Part model, mm, in its own coordinate system. A direction names the side the tool comes from. Round coordinates to 2 decimals unless told otherwise and drop trailing zeros. Order: outer loops, then holes, each group sorted by start corner. A loop starts at its lowest first (then second) coordinate and runs counter-clockwise, first axis right, second up. Notation, with made-up numbers: (89.5, -16.75) -> (134.5, -16.75) arc R29 ccw to (134.5, 4.25) -> close; hole circle Ø8 at (-7, 64.5). An arc over 180 degrees is marked (long way). Answer as a JSON object with one key per item and string values. Group by question number.
```python
from build123d import *

# Parameters (mm, degrees)
F0_W     = 105
F0_H     = 85
F0_W_2   = 72
F0_H_2   = 40
F1_ANGLE = 48


with BuildPart() as f1:
    # F0 (on Front) → F1 (revolve)
    with BuildSketch(Plane.XZ):
        Rectangle(F0_W, F0_H)
        with Locations((0, 12.5)):
            Rectangle(F0_W_2, F0_H_2, mode=Mode.SUBTRACT)
    revolve(axis=Axis((0, 0, -42.5), (-1, 0, 0)), revolution_arc=F1_ANGLE)


solid = f1.part
```
Q1. Band-saw the part on C-C (y = 40). List the corners of the cut face in (x, z), plus the area to 3 significant figures.
Q2. Band-saw the part on D-D (z = 17). List the corners of the cut face in (x, y), plus the area to 3 significant figures.
Q3. Two-plate mould, pull along Z, no slides. Class faces 1 (the cylindrical face through (0.73, 34.12, 35.35)), 2 (the flat face through (-36, 22, 7)), 3 (the flat face through (-52.5, 25, 10)), 4 (the cylindrical face through (0.504, 30.103, 26.194)): +Z half, -Z half, draft (parallel to the pull), parting line (faces both ways), or undercut.
Q4. Which spindle directions (+Z, -Z, +X, -X, +Y, -Y) get a long thin tool onto all of the face, cutting with end or side? Do faces 5 (the flat face through (-1, 0, -9)), 6 (the cylindrical face through (0.504, 14.048, -10.443)). Say none if no direction does.
Q5. Wall check: line 1 (X direction, y = 26, z = 20.5); line 2 (Y direction, x = -14.5, z = 13.5); line 3 (Y direction, x = -42, z = 12). Give the ranges that are in metal, low to high. Write a range as [from, to].
Q6. Band-saw the part on A-A (x = 34.5). List the corners of the cut face in (y, z), plus the area to 3 significant figures.
Q7. Drop flat-ended pins along their axis: pin 1 Ø10 at (y, z) = (25, -32) entering from -X; pin 2 Ø3 at (x, y) = (-7.5, 14.5) entering from -Z; pin 3 Ø10 at (x, z) = (41.5, -10.5) entering from +Y; pin 4 Ø2 at (x, y) = (-9, 41) entering from +Z. Give the stop position or say it passes through.
Q8. Band-saw the part on B-B (z = 6). List the corners of the cut face in (x, y).
Completed:
{
 "1": {"outline": "(-52.5, -6.48) -> (-36, -6.48) -> (-36, 20.94) -> (36, 20.94) -> (36, -6.48) -> (52.5, -6.48) -> (52.5, 32.5) -> (-52.5, 32.5) -> close", "area": "2,120 mm2"},
 "2": {"outline": "(-52.5, 0) -> (-36, 0) -> (-36, 45.66) -> (36, 45.66) -> (36, 0) -> (52.5, 0) -> (52.5, 60.7) -> (-52.5, 60.7) -> close", "area": "3,090 mm2"},
 "3": {"face 1": "+Z half", "face 2": "undercut", "face 3": "draft", "face 4": "undercut"},
 "4": {"face 5": "+Z, -Z, +X, -X, -Y", "face 6": "+Y"},
 "5": {"line 1": "[-52.5, -36], [36, 52.5]", "line 2": "[49.89, 62.19]", "line 3": "[0, 60.53]"},
 "6": {"outline": "(0, -42.5) -> (26.01, -19.08) arc R35 ccw to (0, -7.5) -> close; (0, 32.5) arc R75 cw to (55.74, 7.68) -> (63.17, 14.38) arc R85 ccw to (0, 42.5) -> close", "area": "1,180 mm2"},
 "7": {"pin 1": "through", "pin 2": "z = -30.79", "pin 3": "y = 41.09", "pin 4": "z = 32.5"},
 "8": {"outline": "(-52.5, 0) -> (-36, 0) -> (-36, 53.86) -> (-52.5, 53.86) -> close; (36, 0) -> (52.5, 0) -> (52.5, 53.86) -> (36, 53.86) -> close"}
}
